Source: CAD feature listing. Evaluate the final solid. Frame: model axes, mm. A direction names the side the tool comes from. Give positions to 0.01 mm unless a question says otherwise; leave off trailing zeros. Order: outer loops, then holes, each group sorted by start corner. A loop starts at its lowest first (then second) coordinate and runs counter-clockwise, first axis right, second up. Notation, with made-up numbers: (16, -7) -> (70, -7) arc R22 ccw to (70, 9) -> close; hole circle Ø9 at (-11.5, 58.25). An arc over 180 degrees is marked (long way). Answer in a Markdown table with one row per item.
```python
from build123d import *

# Parameters (mm, degrees)
SKETCH1_W           = 30
SKETCH1_H           = 30
BOSS_EXTRUDE1_DEPTH = 10
SKETCH2_R           = 9.6
SKETCH2_R_2         = 9.55
CUT_EXTRUDE1_DEPTH  = 7
SKETCH3_R           = 4
CUT_EXTRUDE2_DEPTH  = 7
SKETCH4_R           = 2
CUT_EXTRUDE3_DEPTH  = 10
CIRPATTERN1_COUNT   = 4


with BuildPart() as part:
    # Sketch1 → Boss-Extrude1 (new body)
    with BuildSketch(Plane(origin=(0, 0, 0), x_dir=(1, 0, 0), z_dir=(0, 1, 0))):
        Rectangle(SKETCH1_W, SKETCH1_H)
    extrude(amount=BOSS_EXTRUDE1_DEPTH)

    # Sketch2 → Cut-Extrude1 (cut)
    with BuildSketch(Plane(origin=(0, 10, 0), x_dir=(1, 0, 0), z_dir=(0, 1, 0))):
        Circle(SKETCH2_R)
        Circle(SKETCH2_R_2, mode=Mode.SUBTRACT)
    extrude(amount=-CUT_EXTRUDE1_DEPTH, mode=Mode.SUBTRACT)

    # Sketch3 → Cut-Extrude2 (cut)
    with BuildSketch(Plane(origin=(0, 10, 0), x_dir=(1, 0, 0), z_dir=(0, 1, 0))):
        Circle(SKETCH3_R)
    extrude(amount=-CUT_EXTRUDE2_DEPTH, mode=Mode.SUBTRACT)

    # Sketch4 → Cut-Extrude3 (cut)
    with BuildSketch(Plane(origin=(0, 10, 0), x_dir=(1, 0, 0), z_dir=(0, 1, 0))):
        with Locations((10.792349727, 10.987509758)):
            Circle(SKETCH4_R)
    cut_extrude3 = extrude(amount=-CUT_EXTRUDE3_DEPTH, mode=Mode.SUBTRACT)

    # CirPattern1: Cut-Extrude3 ×4 about axis
    cirpattern1_axis = Axis((0, 0, 0), (0, 1, 0))
    for i in range(1, CIRPATTERN1_COUNT):
        add(cut_extrude3.rotate(cirpattern1_axis, i * 360 / CIRPATTERN1_COUNT), mode=Mode.SUBTRACT)


solid = part.part
```
(1) First-contact query: pin 1 Ø3.5 at (x, z) = (-10.79, 10.99) entering from +Y; pin 2 Ø2.5 at (x, z) = (-2, -1.5) entering from +Y. Flat tips, straight axial feed; report the tip coordinate or a pass-through.
A:
| item | result |
|---|---|
| pin 1 | passes through |
| pin 2 | stops at y = 3 |
(2) Section query A-A (z = 0). Return the cut outline in (x, y).
A:
| item | result |
|---|---|
| outline | (-15, 0) -> (15, 0) -> (15, 10) -> (9.6, 10) -> (9.6, 3) -> (9.55, 3) -> (9.55, 10) -> (4, 10) -> (4, 3) -> (-4, 3) -> (-4, 10) -> (-9.55, 10) -> (-9.55, 3) -> (-9.6, 3) -> (-9.6, 10) -> (-15, 10) -> close |
(3) Ray query, probe 1 along X at (y, z) = (4, 10.25); probe 2 along X at (y, z) = (7.25, -10); probe 3 along Y at (x, z) = (1, 1.25). Return the intervals inside material, ascending.
A:
| item | result |
|---|---|
| probe 1 | x = -15 to -12.65, -8.93 to 9.06, 12.91 to 15 |
| probe 2 | x = -15 to -12.82, -9.15 to 9.05, 12.53 to 15 |
| probe 3 | y = 0 to 3 |
(4) Section query D-D (x = -12). Return the cut outline in (y, z).
A:
| item | result |
|---|---|
| outline | (0, -15) -> (10, -15) -> (10, -12.52) -> (0, -12.52) -> close; (0, -9.07) -> (10, -9.07) -> (10, 9.39) -> (0, 9.39) -> close; (0, 12.58) -> (10, 12.58) -> (10, 15) -> (0, 15) -> close |
(5) Pull-direction query (Z, two-part tool) for faces 1 (the flat face through (15, 5, 0)), 2 (the flat face through (0, 5, 15)), 3 (the cylindrical face through (11.59, 5.07, 12.7)); classes: +Z half, -Z half, draft (parallel to the pull), parting line (faces both ways), or undercut.
A:
| item | result |
|---|---|
| face 1 | draft |
| face 2 | +Z half |
| face 3 | undercut |
(6) Access query for faces 4 (the flat face through (2, 10, 4)), 5 (the flat face through (0, 3, 0)). Directions: +Z, -Z, +X, -X, +Y, -Y. A direction counts if a zero-diameter tool reaches every point of the face in a straight line with its end or side. Return the directions, or none.
A:
| item | result |
|---|---|
| face 4 | +Z, -Z, +X, -X, +Y |
| face 5 | +Y |
(7) Section query C-C (x = 0). Return the cut outline in (y, z), plus the area to 3 significant figures.
A:
| item | result |
|---|---|
| outline | (0, -15) -> (10, -15) -> (10, -9.6) -> (3, -9.6) -> (3, -9.55) -> (10, -9.55) -> (10, -4) -> (3, -4) -> (3, 4) -> (10, 4) -> (10, 9.55) -> (3, 9.55) -> (3, 9.6) -> (10, 9.6) -> (10, 15) -> (0, 15) -> close |
| area | 243 mm^2 |
(8) Section query B-B (y = 9.5). Return the cut outline in (x, z), plus the area to 3 significant figures.
A:
| item | result |
|---|---|
| outline | (-15, -15) -> (15, -15) -> (15, 15) -> (-15, 15) -> close; circle Ø19.1 at (0, 0); hole circle Ø4 at (-10.99, -10.79); hole circle Ø4 at (-10.79, 10.99); hole circle Ø19.2 at (0, 0); hole circle Ø8 at (0, 0); hole circle Ø4 at (10.79, -10.99); hole circle Ø4 at (10.99, 10.79) |
| area | 796 mm^2 |
